Autodesk Inventor part; units mm, degrees
ref_plane "YZ Plane" through (0, 0, 0) normal (1, 0, 0) x (0, 1, 0)
ref_plane "XZ Plane" through (0, 0, 0) normal (0, 1, 0) x (-1, 0, 0)
ref_plane "XY Plane" through (0, 0, 0) normal (0, 0, 1) x (1, 0, 0)
sketch "Sketch1" plane through (0, 0, 0) normal (0, 1, 0) x (-1, 0, 0)
  arc A0 (10, 0) -> (6.8806, 7.2566) centre (0, 0) ccw
  arc A1 (151.2194, 7.2566) -> (148.1, 0.0154) centre (158.1, 0) ccw
  arc A2 (29.7625, 6.9475) -> (26.6431, 14.2041) centre (19.7625, 6.9475) ccw
  arc A3 (131.4569, 14.2041) -> (128.3375, 6.9475) centre (138.3375, 6.9475) ccw
  arc A4 (72.1694, 62.2184) -> (85.9306, 62.2184) centre (79.05, 69.475) ccw
  circle A5 centre (79.05, 64.475) radius 1
  circle A6 centre (133.744, 8.9222) radius 1
  circle A7 centre (24.356, 8.9222) radius 1
  line L0 (26.6431, 14.2041) -> (72.1694, 62.2184)
  line L1 (85.9306, 62.2184) -> (131.4569, 14.2041)
  line L2 (128.3375, 6.9475) -> (29.7625, 6.9475)
  line L3 (6.8806, 7.2566) -> (72.1694, 76.1134)
  line L4 (85.9306, 76.1134) -> (151.2194, 7.2566)
  line L5 (148.1, 0.0154) -> (10, 0)
  arc A8 (72.1694, 76.1134) -> (85.9306, 76.1134) centre (79.05, 83.37) ccw
  line L6 (14.0684, 2.4018) -> (17.5684, 2.4018)
  line L7 (17.5684, 2.4018) -> (17.5684, 4.4018)
  line L8 (17.5684, 4.4018) -> (14.0684, 4.4018)
  line L9 (14.0684, 4.4018) -> (14.0684, 2.4018)
  line L10 (77.3084, 2.4018) -> (80.8084, 2.4018)
  line L11 (80.8084, 2.4018) -> (80.8084, 4.4018)
  line L12 (80.8084, 4.4018) -> (77.3084, 4.4018)
  line L13 (77.3084, 4.4018) -> (77.3084, 2.4018)
  line L14 (140.5484, 2.4018) -> (144.0484, 2.4018)
  line L15 (144.0484, 2.4018) -> (144.0484, 4.4018)
  line L16 (144.0484, 4.4018) -> (140.5484, 4.4018)
  line L17 (140.5484, 4.4018) -> (140.5484, 2.4018)
  line L18 (16.2824, 8.7713) -> (18.6906, 11.3111)
  line L19 (18.6906, 11.3111) -> (17.2392, 12.6872)
  line L20 (17.2392, 12.6872) -> (14.831, 10.1474)
  line L21 (14.831, 10.1474) -> (16.2824, 8.7713)
  line L22 (43.688, 37.6746) -> (46.0962, 40.2145)
  line L23 (46.0962, 40.2145) -> (44.6449, 41.5906)
  line L24 (44.6449, 41.5906) -> (42.2367, 39.0508)
  line L25 (42.2367, 39.0508) -> (43.688, 37.6746)
  line L26 (71.0937, 66.578) -> (73.5019, 69.1178)
  line L27 (73.5019, 69.1178) -> (72.0506, 70.4939)
  line L28 (72.0506, 70.4939) -> (69.6424, 67.9541)
  line L29 (69.6424, 67.9541) -> (71.0937, 66.578)
  line L30 (143.2789, 10.1369) -> (140.8707, 12.6767)
  line L31 (140.8707, 12.6767) -> (139.4194, 11.3006)
  line L32 (139.4194, 11.3006) -> (141.8276, 8.7608)
  line L33 (141.8276, 8.7608) -> (143.2789, 10.1369)
  line L34 (115.941, 38.9688) -> (113.5329, 41.5086)
  line L35 (113.5329, 41.5086) -> (112.0815, 40.1325)
  line L36 (112.0815, 40.1325) -> (114.4897, 37.5927)
  line L37 (114.4897, 37.5927) -> (115.941, 38.9688)
  line L38 (88.6032, 67.8006) -> (86.195, 70.3404)
  line L39 (86.195, 70.3404) -> (84.7437, 68.9643)
  line L40 (84.7437, 68.9643) -> (87.1519, 66.4245)
  line L41 (87.1519, 66.4245) -> (88.6032, 67.8006)
  point P0 (151.2194, 7.2566)
  point P1 (85.9306, 76.1134)
  point P2 (29.7625, 6.9475)
  point P3 (131.4569, 14.2041)
extrude "Extrusion1" add sketch "Sketch1" along normal blind 4
properties part number "aab_camera_face"
Work out the finished part from the listing and answer in its coordinate system (mm). A direction names the side the tool comes from. Give positions to 0.01 mm unless a question says otherwise; leave off trailing zeros. Order: outer loops, then holes, each group sorted by start corner. A loop starts at its lowest first (then second) coordinate and runs counter-clockwise, first axis right, second up. Notation, with made-up numbers: (60.5, 61) -> (69.5, 61) arc R15 ccw to (69.5, 87) -> close; hole circle Ø10 at (-37, 61.5). An arc over 180 degrees is marked (long way). Answer as a JSON object with one key per item and string values. Group by question number.
1. A tool of negligible diameter and unlimited length cuts with its end or side. For faces 1 (the flat face through (-16, 2, 2.402)), 2 (the flat face through (-84, 0, 4)), from which of +Z, -Z, +X, -X, +Y, -Y can it reach the whole face along a straight path? Write none if from no direction.
2. Consider line 1 along Z through (x, y) = (-79.05, 2.85) (1 decimal); line 2 along Z through (x, y) = (-16.5, 2.9); line 3 along Z through (x, y) = (-44.5, 0.55). Determine where each line is inside the solid, lowest interval first. Write a range as [from, to].
3. Section B-B on y = 1.4 is taken. Count the separate pieces of the cut face and the enclosed holes in it, plus the area to 3 significant figures.
4. Flat-ended cylindrical pins translate along their axes: pin 1 Ø1.8 at (x, y) = (-16, 2.5) entering from +Z; pin 2 Ø1 at (y, z) = (3, 3.5) entering from +X; pin 3 Ø1 at (x, y) = (-78.5, 2) entering from -Z. Find the tip coordinate at first contact, or state that the pin passes through.
5. Section A-A on x = -92 is taken. Determine the outline of the cut face in (y, z).
6. The mould has two halves that part along Z. Classify faces 3 (the cylindrical face through (-28.927, 1.972, 10.949)), 4 (the flat face through (-118.118, 1.972, 42.167)), 5 (the cylindrical face through (-9.165, 1.972, 4.001)), 6 (the flat face through (-16, 2, 4.402)): released by +Z, released by -Z, zero draft, split by the parting line, or undercut.
Result sheet:
{
 "1": {"face 1": "+Y, -Y", "face 2": "+Z, -Z, +X, -X, -Y"},
 "2": {"line 1": "z = [0, 2.4], [4.4, 6.9], [59.5, 63.5], [65.5, 73.4]", "line 2": "z = [0, 2.4], [4.4, 9], [11.91, 17.4]", "line 3": "z = [0, 6.95], [33.04, 38.53], [41.44, 46.93]"},
 "3": {"separate pieces": "1", "enclosed holes": "13", "area": "2,810 mm^2"},
 "4": {"pin 1": "stops at z = 17.82", "pin 2": "stops at x = -9.17", "pin 3": "stops at z = 0.01"},
 "5": {"outline": "(0, 0.01) -> (4, 0.01) -> (4, 6.95) -> (0, 6.95) -> close; (0, 55.82) -> (4, 55.82) -> (4, 69.71) -> (0, 69.71) -> close"},
 "6": {"face 3": "undercut", "face 4": "released by +Z", "face 5": "released by -Z", "face 6": "undercut"}
}
